Verification items for the finished model (mm, model axes). A direction names the side the tool comes from. Coordinates: 2 decimals unless noted, no trailing zeros. Order: outer loops, then holes, each group sorted by start corner. A loop starts at its lowest first (then second) coordinate and runs counter-clockwise, first axis right, second up. Notation, with made-up numbers: M 31,14.25 L 60,14.25 A23 ccw 60,51.25 Z; hole C -38,59 d7. An arc over 180 degrees is marked long. Return JSON: item names as keys, results as strings.
```python
from build123d import *

# Parameters (mm, degrees)
F0_R      = 2
F0_W      = 27.5
F0_H      = 48
F1_DEPTH  = 1
F0_W_2    = 69
F0_H_2    = 99.5
F2_DEPTH  = 40
F3_W      = 54
F3_H      = 59.5
F3_R      = 2
F3_W_2    = 27.5
F3_H_2    = 48
F4_DEPTH  = 30
F5_W      = 48.8
F5_H      = 16
F6_DEPTH  = 40.001
F7_R      = 2.25
F8_DEPTH  = 20.201
F9_DEPTH  = 1
F11_DEPTH = 40.001


with BuildPart() as f1:
    # F0 (on Top) → F1 (new body)
    with BuildSketch(Plane.XY):
        Polygon((7.5751999344, 18.5791517273), (-21.0248000656, 18.5791517273), (-31.2248000656, -11.1708482727), (-21.0248000656, -40.9208482727), (7.5751999344, -40.9208482727), (17.7751999344, -11.1708482727), align=None)
        with Locations((-26.7248000656, -11.1708482727)):
            Circle(F0_R, mode=Mode.SUBTRACT)
        with Locations((-6.7248000656, -11.1708482727)):
            Rectangle(F0_W, F0_H, mode=Mode.SUBTRACT)
        with Locations((13.2751999344, -11.1708482727)):
            Circle(F0_R, mode=Mode.SUBTRACT)
    extrude(amount=F1_DEPTH)

    # F0 (on Top) → F2 (join)
    with BuildSketch(Plane.XY):
        with Locations((-6.7248000656, -11.1708482727)):
            Rectangle(F0_W_2, F0_H_2)
        Polygon((-31.2248000656, -11.1708482727), (-21.0248000656, 18.5791517273), (7.5751999344, 18.5791517273), (17.7751999344, -11.1708482727), (7.5751999344, -40.9208482727), (-21.0248000656, -40.9208482727), align=None, mode=Mode.SUBTRACT)
        Polygon((7.5751999344, 18.5791517273), (-21.0248000656, 18.5791517273), (-31.2248000656, -11.1708482727), (-21.0248000656, -40.9208482727), (7.5751999344, -40.9208482727), (17.7751999344, -11.1708482727), align=None)
        with Locations((-26.7248000656, -11.1708482727)):
            Circle(F0_R, mode=Mode.SUBTRACT)
        with Locations((-6.7248000656, -11.1708482727)):
            Rectangle(F0_W, F0_H, mode=Mode.SUBTRACT)
        with Locations((13.2751999344, -11.1708482727)):
            Circle(F0_R, mode=Mode.SUBTRACT)
    extrude(amount=-F2_DEPTH)

    # F3 (on face) → F4 (cut)
    with BuildSketch(Plane(origin=(0, 0, -40), x_dir=(1, 0, 0), z_dir=(0, 0, -1))):
        with Locations((-6.7248000656, 11.1708482727)):
            Rectangle(F3_W, F3_H)
        with Locations((-26.7248000656, 11.1708482727)):
            Circle(F3_R, mode=Mode.SUBTRACT)
        with Locations((-6.7248000656, 11.1708482727)):
            Rectangle(F3_W_2, F3_H_2, mode=Mode.SUBTRACT)
        with Locations((13.2751999344, 11.1708482727)):
            Circle(F3_R, mode=Mode.SUBTRACT)
    extrude(amount=-F4_DEPTH, mode=Mode.SUBTRACT)

    # F5 (on face) → F6 (cut, through all)
    with BuildSketch(Plane.XY):
        with Locations((-16.8248000656, -52.9208482727)):
            Rectangle(F5_W, F5_H)
        with Locations((-16.8248000656, 30.5791517273)):
            Rectangle(F5_W, F5_H)
    extrude(amount=-F6_DEPTH, mode=Mode.SUBTRACT)

    # F7 (on face) → F8 (cut, through all)
    with BuildSketch(Plane(origin=(7.5751999344, 0, 0), x_dir=(0, -1, 0), z_dir=(-1, 0, 0))):
        with Locations((52.9208482727, -10)):
            Circle(F7_R)
        with Locations((52.9208482727, -30)):
            Circle(F7_R)
        with Locations((-30.5791517273, -10)):
            Circle(F7_R)
        with Locations((-30.5791517273, -30)):
            Circle(F7_R)
    extrude(amount=-F8_DEPTH, mode=Mode.SUBTRACT)

    # F9 (cut): a face of the model
    f9_faces = [f1.faces().sort_by_distance(p)[0] for p in [
        (-6.7248000656, 17.8083566832, 1),
    ]]
    extrude(f9_faces, amount=-F9_DEPTH, mode=Mode.SUBTRACT)

    # F10 (on face) → F11 (cut, through all)
    with BuildSketch(Plane(origin=(0, 0, -40), x_dir=(1, 0, 0), z_dir=(0, 0, -1))):
        with BuildLine():
            ThreePointArc((-41.2248000656, 39.9208482727), (-39.7603339715, 43.4563821787), (-36.2248000656, 44.9208482727))
            Line((-36.2248000656, 44.9208482727), (-41.2248000656, 44.9208482727))
            Line((-41.2248000656, 44.9208482727), (-41.2248000656, 39.9208482727))
        make_face()
        with BuildLine():
            ThreePointArc((-36.2248000656, -22.5791517273), (-39.7603339715, -21.1146856332), (-41.2248000656, -17.5791517273))
            Line((-41.2248000656, -17.5791517273), (-41.2248000656, -22.5791517273))
            Line((-41.2248000656, -22.5791517273), (-36.2248000656, -22.5791517273))
        make_face()
    extrude(amount=-F11_DEPTH, mode=Mode.SUBTRACT)


solid = f1.part
```
Q1. Cross-section at B-B, the plane z = -21.5. Record the boundary of the cut face in (x, y), and give its area (3 significant figures).
Values:
{"outline": "M -41.22,-39.92 A5 ccw -36.22,-44.92 L 7.58,-44.92 L 7.58,-60.92 L 27.78,-60.92 L 27.78,38.58 L 7.58,38.58 L 7.58,22.58 L -36.22,22.58 A5 ccw -41.22,17.58 Z; hole M -33.72,-40.92 L 20.28,-40.92 L 20.28,18.58 L -33.72,18.58 Z", "area": "2,080 mm^2"}
Q2. Cross-section at C-C, the plane y = -16.5. Record the boundary of the cut face in (x, z), and give its area (3 significant figures).
Values:
{"outline": "M -41.22,-40 L -33.72,-40 L -33.72,-10 L -20.47,-10 L -20.47,0 L -41.22,0 Z; M 7.03,-10 L 20.28,-10 L 20.28,-40 L 27.78,-40 L 27.78,0 L 7.03,0 Z", "area": "865 mm^2"}
Q3. Tool access check on faces 1 (the face through (-15, 22.579, -20)), 2 (the face through (7.575, -53, -20)), 3 (the face through (-7, -40.921, -25)), 4 (the face through (-7, 12.829, -5)). Record the directions out of +Z, -Z, +X, -X, +Y, -Y that give a thin tool (end or side, any length) a straight path to the whole face; none if there is none.
Values:
{"face 1": "+Z, -Z, -X, +Y", "face 2": "+Z, -Z, -X, -Y", "face 3": "-Z", "face 4": "+Z, -Z"}
Q4. Cross-section at A-A, the plane z = -30. Record the boundary of the cut face in (x, y).
Values:
{"outline": "M -41.22,-39.92 A5 ccw -36.22,-44.92 L 7.58,-44.92 L 7.58,-50.67 L 27.78,-50.67 L 27.78,28.33 L 7.58,28.33 L 7.58,22.58 L -36.22,22.58 A5 ccw -41.22,17.58 Z; M 7.58,-60.92 L 27.78,-60.92 L 27.78,-55.17 L 7.58,-55.17 Z; M 7.58,32.83 L 27.78,32.83 L 27.78,38.58 L 7.58,38.58 Z; hole M -33.72,-40.92 L 20.28,-40.92 L 20.28,18.58 L -33.72,18.58 Z"}
Q5. Material ranges on line 1 along X through (y, z) = (-13, -38); line 2 along Y through (x, z) = (-16.5, -26); line 3 along Y through (x, z) = (10, -27), recorded low to high.
Values:
{"line 1": "-41.22 to -33.72, 20.28 to 27.78", "line 2": "-44.92 to -40.92, 18.58 to 22.58", "line 3": "-60.92 to -40.92, 18.58 to 38.58"}
Q6. Draft check along Y on faces 5 (the face through (-41.225, -12, -20)), 6 (the face through (-39.721, 21.153, -20.28)), 7 (the face through (-20.475, -12, -5)), 8 (the face through (-15, -44.921, -20)). Enter one of: pulls with the +Y half, pulls with the -Y half, needs draft (parallel to the pull), parting line crosses it, or undercut.
Values:
{"face 5": "needs draft", "face 6": "pulls with the +Y half", "face 7": "undercut", "face 8": "pulls with the -Y half"}
Q7. Go/stop test with flat-tipped pins: pin 1 (6 mm diameter, centred on y = -52.92, z = -30, fed in from -X); pin 2 (15 mm diameter, centred on x = -20, z = -27.5, fed in from -Y); pin 3 (11 mm diameter, centred on x = 0, z = -2.5, fed in from +Y). Record where each tip stops, or that it passes through.
Values:
{"pin 1": "x = 7.58", "pin 2": "y = -44.92", "pin 3": "y = 22.58"}
Q8. Cross-section at D-D, the plane x = -12.5. Record the boundary of the cut face in (y, z), and give its area (3 significant figures).
Values:
{"outline": "M -44.92,-40 L -40.92,-40 L -40.92,-10 L -35.17,-10 L -35.17,0 L -44.92,0 Z; M 12.83,-10 L 18.58,-10 L 18.58,-40 L 22.58,-40 L 22.58,0 L 12.83,0 Z", "area": "435 mm^2"}
